The listing builds one solid part. Answer for the finished solid, in the listing's coordinates (mm). A direction names the side the tool comes from. Give positions to 0.01 mm unless a question says otherwise; leave off trailing zeros. Write each loop counter-clockwise with the first axis right and the second up, starting at its lowest first coordinate (ties: lowest second). Pieces come first, ordered by that corner, then holes. Notation, with made-up numbers: (60.5, 68.25) - (69.5, 68.25) arc R10 cw to (69.5, 74.25) - close; hole circle Ø2 at (-40, -6). An arc over 180 degrees is marked (long way). Answer as CSV lines item,"result". Start each with the question number.
(1) Find section C-C (y = -1.2). Write down the section's boundary in (x, z) (3 decimals), then the cut area to 3 significant figures.
(2) Straight lines are drawn through the part: probe 1 along X at (y, z) = (-2.8, -19); probe 2 along X at (y, z) = (-4.4, 4); probe 3 along Z at (x, y) = (-2, -0.3). For each, find the intervals that lie inside material, in ascending order.
(3) For a pull along Z with two mould halves and no side action, classify faces 1 (the face through (-2.646, -3.589, -11.667)), 2 (the face through (0, -2, 19.05)), 3 (the face through (-0.86, -2.348, -25.385)), 4 (the face through (4.7, -3.6, -15.9)) as pulls with the +Z half, pulls with the -Z half, needs draft (parallel to the pull), parting line crosses it, or undercut.
(4) Find section A-A (z = 0). Write down the section's boundary in (x, y) (1 decimal), then the cut area to 3 significant figures.
(5) Each of these flat-tipped pins is pushed along its axis until it touches: pin 1 Ø2.5 at (x, y) = (6, -3) entering from -Z; pin 2 Ø5 at (x, z) = (0, -16.66) entering from -Y; pin 3 Ø2 at (x, y) = (14.5, -2.5) entering from -Z; pin 4 Ø3 at (x, z) = (18, 0.5) entering from -Y. Where does it stop, or does it pass through?
(6) Find section D-D (x = 15.5). Write down the section's boundary in (y, z).
(7) For faces 5 (the face through (0, -4, 15.875)), 6 (the face through (11.26, -2.35, 8.47)), determine the directions among +Z, -Z, +X, -X, +Y, -Y from which every point of the face is accessible in a straight line to the end or side of a thin tool.
(8) Find section B-B (x = 0). State how many separate pieces and enclosed holes the cut face has, then the cut area to 3 significant figures.
from build123d import *

# Parameters (mm, degrees)
F0_R     = 25.4
F0_R_2   = 3.175
F0_R_3   = 8
F1_DEPTH = 4.7625
F2_W     = 50.561215
F2_H     = 14.34433
F3_DEPTH = 25.4
F5_DEPTH = 2.38125


with BuildPart() as f1:
    # F0 (on Front) → F1 (new body)
    with BuildSketch(Plane.XZ):
        Circle(F0_R)
        with Locations((0, -16.6624)):
            Circle(F0_R_2, mode=Mode.SUBTRACT)
        Circle(F0_R_3, mode=Mode.SUBTRACT)
        with Locations((-14.430062, 8.3312)):
            Circle(F0_R_2, mode=Mode.SUBTRACT)
        with Locations((14.430062, 8.3312)):
            Circle(F0_R_2, mode=Mode.SUBTRACT)
    extrude(amount=F1_DEPTH)

    # F2 (on face) → F3 (cut)
    with BuildSketch(Plane.XZ.offset(4.7625)):
        with Locations((0.75591, 26.222165)):
            Rectangle(F2_W, F2_H)
    extrude(amount=-F3_DEPTH, mode=Mode.SUBTRACT)

    # F4 (on face) → F5 (cut)
    with BuildSketch(Plane.XZ.offset(4.7625)):
        with BuildLine():
            ThreePointArc((-3.646079, -10.497322), (-9.623707, -5.55625), (-10.913987, 2.091064))
            ThreePointArc((-10.913987, 2.091064), (-11.409826, 3.527057), (-12.900289, 3.821078))
            ThreePointArc((-12.900289, 3.821078), (-16.190201, 3.905896), (-18.639619, 6.103863))
            ThreePointArc((-18.639619, 6.103863), (-20.156405, 6.905634), (-21.458089, 5.788007))
            ThreePointArc((-21.458089, 5.788007), (-19.247415, -11.1125), (-5.716484, -21.477254))
            ThreePointArc((-5.716484, -21.477254), (-4.097748, -20.908775), (-4.033709, -19.194315))
            ThreePointArc((-4.033709, -19.194315), (-4.712495, -15.974073), (-3.140994, -13.082517))
            ThreePointArc((-3.140994, -13.082517), (-2.650392, -11.644727), (-3.646079, -10.497322))
        make_face()
        with BuildLine():
            ThreePointArc((-7.267908, 8.406258), (0, 11.1125), (7.267908, 8.406258))
            ThreePointArc((7.267908, 8.406258), (8.759433, 8.11767), (9.759295, 9.261439))
            ThreePointArc((9.759295, 9.261439), (10.905182, 11.533797), (13.057597, 12.891655))
            ThreePointArc((13.057597, 12.891655), (14.126157, 14.572961), (12.618408, 15.875))
            Line((12.618408, 15.875), (-12.618408, 15.875))
            ThreePointArc((-12.618408, 15.875), (-14.126157, 14.572961), (-13.057597, 12.891655))
            ThreePointArc((-13.057597, 12.891655), (-10.905182, 11.533797), (-9.759295, 9.261439))
            ThreePointArc((-9.759295, 9.261439), (-8.759433, 8.11767), (-7.267908, 8.406258))
        make_face()
        with BuildLine():
            ThreePointArc((10.913987, 2.091064), (9.623707, -5.55625), (3.646079, -10.497322))
            ThreePointArc((3.646079, -10.497322), (2.650392, -11.644727), (3.140994, -13.082517))
            ThreePointArc((3.140994, -13.082517), (4.712495, -15.974073), (4.033709, -19.194315))
            ThreePointArc((4.033709, -19.194315), (4.097748, -20.908775), (5.716484, -21.477254))
            ThreePointArc((5.716484, -21.477254), (19.247415, -11.1125), (21.458089, 5.788007))
            ThreePointArc((21.458089, 5.788007), (20.156405, 6.905634), (18.639619, 6.103863))
            ThreePointArc((18.639619, 6.103863), (16.190201, 3.905896), (12.900289, 3.821078))
            ThreePointArc((12.900289, 3.821078), (11.409826, 3.527057), (10.913987, 2.091064))
        make_face()
    extrude(amount=-F5_DEPTH, mode=Mode.SUBTRACT)


solid = f1.part
Result set:
1,outline,"(-16.801, 19.05) arc R25.4 ccw (long way) to (16.801, 19.05) - close; hole circle Ø6.35 at (-14.43, 8.331); hole circle Ø16 at (0, 0); hole circle Ø6.35 at (0, -16.662); hole circle Ø6.35 at (14.43, 8.331)"
1,area,"1,580 mm^2"
2,probe 1,"-16.86 to -11.53, -4.15 to -2.15, 2.15 to 4.15, 11.53 to 16.86"
2,probe 2,"-25.08 to -21.86, -16.41 to -6.93, 6.93 to 16.41, 21.86 to 25.08"
2,probe 3,"-25.32 to -19.13, -14.2 to -7.75, 7.75 to 19.05"
3,face 1,"undercut"
3,face 2,"pulls with the +Z half"
3,face 3,"parting line crosses it"
3,face 4,"undercut"
4,outline,"(-25.4, -4.8) - (-22.2, -4.8) - (-22.2, -2.4) - (-11.1, -2.4) - (-11.1, -4.8) - (-8, -4.8) - (-8, 0) - (-25.4, 0) - close; (8, -4.8) - (11.1, -4.8) - (11.1, -2.4) - (22.2, -2.4) - (22.2, -4.8) - (25.4, -4.8) - (25.4, 0) - (8, 0) - close"
4,area,"113 mm^2"
5,pin 1,"z = -24.95"
5,pin 2,"through"
5,pin 3,"z = -21.52"
5,pin 4,"y = -2.38"
6,outline,"(-4.76, -20.12) - (0, -20.12) - (0, 5.34) - (-4.76, 5.34) - (-4.76, 3.69) - (-2.38, 3.69) - (-2.38, -15.93) - (-4.76, -15.93) - close; (-4.76, 11.32) - (0, 11.32) - (0, 19.05) - (-4.76, 19.05) - close"
7,face 5,"-Y"
7,face 6,"+Y, -Y"
8,separate pieces,"3"
8,enclosed holes,"0"
8,area,"93.9 mm^2"
